For this review, take the finished solid that the model builds, in its own axes (mm). A direction names the side the tool comes from. Coordinates: 2 decimals unless noted, no trailing zeros. Write each loop counter-clockwise with the first axis right and the second up, starting at its lowest first coordinate (ties: lowest second). Pieces come first, ordered by that corner, then holes.
```python
from build123d import *

# Parameters (mm, degrees)
F0_W     = 79.375
F0_H     = 98.425
F1_DEPTH = 3.175
F2_W     = 3.175
F2_H     = 15.875
F3_DEPTH = 3.176
F4_W     = 12.7
F4_H     = 3.175
F5_DEPTH = 3.176


with BuildPart() as f1:
    # F0 (on Right) → F1 (new body)
    with BuildSketch(Plane.YZ):
        Rectangle(F0_W, F0_H)
    extrude(amount=F1_DEPTH)

    # F2 (on face) → F3 (cut, through all)
    with BuildSketch(Plane.YZ.offset(3.175)):
        with Locations((-38.1, 28.575)):
            Rectangle(F2_W, F2_H)
        with Locations((-38.1, 0)):
            Rectangle(F2_W, F2_H)
        with Locations((-38.1, -28.575)):
            Rectangle(F2_W, F2_H)
        with Locations((38.1, 28.575)):
            Rectangle(F2_W, F2_H)
        with Locations((38.1, -28.575)):
            Rectangle(F2_W, F2_H)
        with Locations((38.1, 0)):
            Rectangle(F2_W, F2_H)
    extrude(amount=-F3_DEPTH, mode=Mode.SUBTRACT)

    # F4 (on face) → F5 (cut, through all)
    with BuildSketch(Plane.YZ.offset(3.175)):
        with Locations((-33.3375, 47.625)):
            Rectangle(F4_W, F4_H)
        with Locations((-11.1125, 47.625)):
            Rectangle(F4_W, F4_H)
        with Locations((11.1125, 47.625)):
            Rectangle(F4_W, F4_H)
        with Locations((33.3375, 47.625)):
            Rectangle(F4_W, F4_H)
    extrude(amount=-F5_DEPTH, mode=Mode.SUBTRACT)


solid = f1.part
```
Q1. Add section B-B (y = 14.5). State the section outline as (x, z) points (1 decimal), then the cut area to 3 significant figures.
Ans:
outline: (0, -49.2) - (3.2, -49.2) - (3.2, 46) - (0, 46) - close
area: 302 mm2
Q2. Draft analysis for pull direction Y (two halves, no side actions). For faces 6 (the flat face through (2, -39.688, -43)), 7 (the flat face through (2, -11, 46.038)), 8 (the flat face through (3.175, -1, 1)), 9 (the flat face through (2, -4.763, 48)), state which applies: +Y half, -Y half, draft (parallel to the pull), parting line (faces both ways), or undercut.
Ans:
face 6: -Y half
face 7: undercut
face 8: draft
face 9: undercut
Q3. Add section A-A (z = -34.5). State the section outline as (x, y) points (1 decimal).
Ans:
outline: (0, -36.5) - (3.2, -36.5) - (3.2, 36.5) - (0, 36.5) - close
Q4. For probe 1 along Y at (x, z) = (0.7, 26); probe 2 along Z at (x, y) = (3, 31), list the stretches that pass through material, from the lowest coordinate up.
Ans:
probe 1: y = -36.51 to 36.51
probe 2: z = -49.21 to 46.04
Q5. Tool access review of faces 1 (the flat face through (2, 11, 46.038)), 2 (the flat face through (2, 38, 36.512)), 3 (the flat face through (2, 33, 46.038)), 4 (the flat face through (2, -36.512, 28)), 5 (the flat face through (2, -33, 46.038)): name each direction out of +Z, -Z, +X, -X, +Y, -Y from which nothing blocks a thin tool from reaching the whole face with its end or side.
Ans:
face 1: +Z, +X, -X
face 2: +X, -X, +Y
face 3: +Z, +X, -X, +Y
face 4: +X, -X, -Y
face 5: +Z, +X, -X, -Y
Q6. Clearance check with flat-ended pins moving along their axes: pin 1 Ø1 at (x, z) = (1.5, -1) entering from +Y; pin 2 Ø1.6 at (x, y) = (2, 9) entering from +Z. State where each tip first meets the part, or that it passes through.
Ans:
pin 1: stops at y = 36.51
pin 2: stops at z = 46.04
